Check sheet for the modelled part. Datum: model origin and axes. Units: mm. Give positions to 0.01 mm unless a question says otherwise; leave off trailing zeros. Order: outer loops, then holes, each group sorted by start corner. A loop starts at its lowest first (then second) coordinate and runs counter-clockwise, first axis right, second up. Notation, with made-up numbers: (87.5, 57) -> (129.5, 57) arc R16 cw to (129.5, 82) -> close; hole circle Ø11 at (11, 66). An arc over 180 degrees is marked (long way). One line per question, with ' | ' between items.
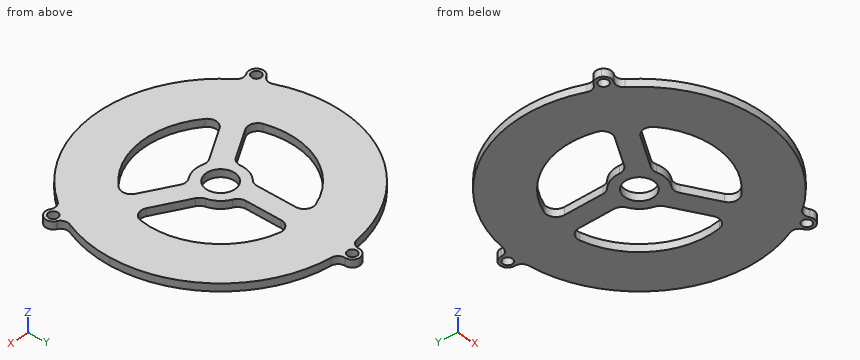
```python
from build123d import *

# Parameters (mm, degrees)
F0_R     = 4.826
F0_R_2   = 1.5875
F1_DEPTH = 2.54
F2_R     = 2.53999


# Not quite as in the source:
# - a fillet or chamfer is up to 0.001 mm smaller than in the source, because OpenCascade refuses the exact size


with BuildPart() as f1:
    # F0 (on Top) → F1 (new body)
    with BuildSketch(Plane.XY):
        with BuildLine():
            ThreePointArc((36.9474511246, -18.3986814852), (40.1785494398, -9.4503857019), (41.275, 0))
            ThreePointArc((41.275, 0), (30.0704516511, 28.2735488133), (2.54, 41.1967720216))
            ThreePointArc((2.54, 41.1967720216), (0, 41.275), (-2.54, 41.1967720216))
            ThreePointArc((-2.54, 41.1967720216), (-35.7451985412, 20.6375), (-36.9474511246, -18.3986814852))
            ThreePointArc((-36.9474511246, -18.3986814852), (-35.7451985412, -20.6375), (-34.4074511246, -22.7980905364))
            ThreePointArc((-34.4074511246, -22.7980905364), (0, -41.275), (34.4074511246, -22.7980905364))
            ThreePointArc((34.4074511246, -22.7980905364), (35.7451985412, -20.6375), (36.9474511246, -18.3986814852))
        make_face()
        with BuildLine():
            ThreePointArc((-16.1831892187, -19.5771393904), (-17.3242054231, -16.864916263), (-15.7477905664, -14.3803663096))
            Line((-15.7477905664, -14.3803663096), (-4.6795539693, -7.9901169308))
            ThreePointArc((-4.6795539693, -7.9901169308), (-3.4772976031, -7.5882063232), (-2.2136295462, -7.6886829322))
            ThreePointArc((-2.2136295462, -7.6886829322), (1.2293114508, -7.9059973664), (4.4437139688, -6.6535259196))
            ThreePointArc((4.4437139688, -6.6535259196), (6.1035441451, -6.1205029783), (7.7945925279, -6.544183326))
            Line((7.7945925279, -6.544183326), (17.8798534353, -12.3669114257))
            ThreePointArc((17.8798534353, -12.3669114257), (19.431886995, -14.6433042701), (18.6198324975, -17.2760480945))
            ThreePointArc((18.6198324975, -17.2760480945), (1.6757275748, -25.3446628917), (-16.1831892187, -19.5771393904))
        make_face(mode=Mode.SUBTRACT)
        Circle(F0_R, mode=Mode.SUBTRACT)
        with BuildLine():
            ThreePointArc((-24.2714127756, -7.4872239098), (-22.786985702, 11.2211087963), (-8.8627054362, 23.8036226729))
            ThreePointArc((-8.8627054362, 23.8036226729), (-5.9433432049, 23.4356601283), (-4.5798672566, 20.8281698388))
            Line((-4.5798672566, 20.8281698388), (-4.5798672566, 8.0476710812))
            ThreePointArc((-4.5798672566, 8.0476710812), (-4.8329306435, 6.8055312224), (-5.5517799678, 5.7614008877))
            ThreePointArc((-5.5517799678, 5.7614008877), (-7.4614502869, 2.8883837376), (-7.9839794556, -0.5216062243))
            ThreePointArc((-7.9839794556, -0.5216062243), (-8.3522831357, -2.2255727936), (-9.5647252713, -3.4782234783))
            Line((-9.5647252713, -3.4782234783), (-19.6499861787, -9.3009515781))
            ThreePointArc((-19.6499861787, -9.3009515781), (-22.3974169907, -9.5068556461), (-24.2714127756, -7.4872239098))
        make_face(mode=Mode.SUBTRACT)
        with BuildLine():
            Line((1.7701327434, 10.0224068043), (1.7701327434, 21.6678630038))
            ThreePointArc((1.7701327434, 21.6678630038), (2.9655299957, 24.1501599162), (5.6515802781, 24.7632720043))
            ThreePointArc((5.6515802781, 24.7632720043), (21.1112581272, 14.1235540955), (25.0458946549, -4.2264832825))
            ThreePointArc((25.0458946549, -4.2264832825), (23.267548628, -6.5707438653), (20.327657823, -6.4478035292))
            Line((20.327657823, -6.4478035292), (9.259421226, -0.0575541504))
            ThreePointArc((9.259421226, -0.0575541504), (8.3102282466, 0.7826751008), (7.7654095141, 1.9272820445))
            ThreePointArc((7.7654095141, 1.9272820445), (6.2321388361, 5.0176136288), (3.5402654867, 7.175132144))
            ThreePointArc((3.5402654867, 7.175132144), (2.2487389906, 8.3460757719), (1.7701327434, 10.0224068043))
        make_face(mode=Mode.SUBTRACT)
        with BuildLine():
            ThreePointArc((-2.54, 41.1967720216), (0, 41.275), (2.54, 41.1967720216))
            Line((2.54, 41.1967720216), (2.54, 46.2767720216))
            Line((2.54, 46.2767720216), (-2.54, 46.2767720216))
            Line((-2.54, 46.2767720216), (-2.54, 41.1967720216))
        make_face()
        with Locations((0, 43.7367720216)):
            Circle(F0_R_2, mode=Mode.SUBTRACT)
        with BuildLine():
            ThreePointArc((-34.4074511246, -22.7980905364), (-35.7451985412, -20.6375), (-36.9474511246, -18.3986814852))
            Line((-36.9474511246, -18.3986814852), (-41.3468601758, -20.9386814852))
            Line((-41.3468601758, -20.9386814852), (-38.8068601758, -25.3380905364))
            Line((-38.8068601758, -25.3380905364), (-34.4074511246, -22.7980905364))
        make_face()
        with Locations((-37.8771556502, -21.8683860108)):
            Circle(F0_R_2, mode=Mode.SUBTRACT)
        with BuildLine():
            Line((41.3468601758, -20.9386814852), (36.9474511246, -18.3986814852))
            ThreePointArc((36.9474511246, -18.3986814852), (35.7451985412, -20.6375), (34.4074511246, -22.7980905364))
            Line((34.4074511246, -22.7980905364), (38.8068601758, -25.3380905364))
            Line((38.8068601758, -25.3380905364), (41.3468601758, -20.9386814852))
        make_face()
        with Locations((37.8771556502, -21.8683860108)):
            Circle(F0_R_2, mode=Mode.SUBTRACT)
    extrude(amount=F1_DEPTH)

    # F2 (radius 2.54 in the source; OpenCascade refuses exactly that, so slightly less here)
    f2_edges = [f1.edges().sort_by_distance(p)[0] for p in [
        (-34.407451, -22.798091, 1.27),
        (-38.80686, -25.338091, 1.27),
        (-41.34686, -20.938681, 1.27),
        (-36.947451, -18.398681, 1.27),
        (34.407451, -22.798091, 1.27),
        (38.80686, -25.338091, 1.27),
        (41.34686, -20.938681, 1.27),
        (36.947451, -18.398681, 1.27),
        (2.54, 41.196772, 1.27),
        (2.54, 46.276772, 1.27),
        (-2.54, 41.196772, 1.27),
        (-2.54, 46.276772, 1.27),
    ]]
    fillet(f2_edges, radius=F2_R)


solid = f1.part
```
Q1. Depth check by flat-ended pin: pin 1 Ø1.9 at (x, y) = (-37.88, -21.87) entering from +Z. Enter the tip coordinate at first touch or a pass-through.
Result sheet:
pin 1: passes through
Q2. Section check C-C (z = 1.15). Count the separate pieces of the cut face and the enclosed holes in it, and give its area (3 significant figures).
Result sheet:
separate pieces: 1 | enclosed holes: 7 | area: 3,870 mm2
Q3. Thickness scan on line 1 (Y direction, x = 0, z = 1.9) (3 decimals); line 2 (X direction, y = 11, z = 1.05); line 3 (X direction, y = 5.5, z = 1.5). Record the ranges inside material, lowest first.
Result sheet:
line 1: y = -41.275 to -25.4, -8.001 to -4.826, 4.826 to 42.149, 45.324 to 46.277 | line 2: x = -39.78 to -22.89, -4.58 to 1.77, 22.89 to 39.78 | line 3: x = -40.91 to -24.8, -5.81 to 5.81, 24.8 to 40.91
Q4. Section check B-B (x = 23). Enter the section's corners in (y, z), and give its area (3 significant figures).
Result sheet:
outline: (-34.27, 0) -> (-6.68, 0) -> (-6.68, 2.54) -> (-34.27, 2.54) -> close; (10.78, 0) -> (34.27, 0) -> (34.27, 2.54) -> (10.78, 2.54) -> close | area: 130 mm2
Q5. Section check D-D (y = -28.5). Enter the section's corners in (x, z).
Result sheet:
outline: (-29.86, 0) -> (29.86, 0) -> (29.86, 2.54) -> (-29.86, 2.54) -> close
Q6. Section check A-A (x = 11). Enter the section's corners in (y, z).
Result sheet:
outline: (-39.78, 0) -> (-22.89, 0) -> (-22.89, 2.54) -> (-39.78, 2.54) -> close; (-8.39, 0) -> (-1.06, 0) -> (-1.06, 2.54) -> (-8.39, 2.54) -> close; (22.89, 0) -> (39.78, 0) -> (39.78, 2.54) -> (22.89, 2.54) -> close
